The model under review builds one solid part; all positions refer to its coordinate system, in mm. Give positions to 0.01 mm unless a question says otherwise; leave off trailing zeros. Loops run counter-clockwise (first coordinate to the right, second up) from the corner with the lowest first, then second, coordinate; pieces in that order, holes last. Notation, with made-up numbers: M 8.25,-10.5 L 30.25,-10.5 A23 cw 30.25,27.5 Z; hole C 70,-39.5 d9. An arc over 180 degrees is marked long. Return JSON: item names as keys, results as strings.
```python
from build123d import *

# Parameters (mm, degrees)
BOSS_EXTRUDE1_DEPTH = 3.5
SKETCH2_R           = 3.5
SKETCH2_W           = 100
SKETCH2_H           = 40
CUT_EXTRUDE1_DEPTH  = 3.5


with BuildPart() as part:
    # Sketch1 → Boss-Extrude1 (new body)
    with BuildSketch(Plane(origin=(0, 0, 0), x_dir=(1, 0, 0), z_dir=(0, 1, 0))):
        with BuildLine():
            Line((-91.7, 73.2), (91.7, 73.2))
            ThreePointArc((91.7, 73.2), (101.953048327, 68.953048327), (106.2, 58.7))
            Line((106.2, 58.7), (106.2, -58.7))
            ThreePointArc((106.2, -58.7), (101.953048327, -68.953048327), (91.7, -73.2))
            Line((91.7, -73.2), (-91.7, -73.2))
            ThreePointArc((-91.7, -73.2), (-101.953048327, -68.953048327), (-106.2, -58.7))
            Line((-106.2, -58.7), (-106.2, 58.7))
            ThreePointArc((-106.2, 58.7), (-101.953048327, 68.953048327), (-91.7, 73.2))
        make_face()
    extrude(amount=BOSS_EXTRUDE1_DEPTH)

    # Sketch2 → Cut-Extrude1 (cut)
    with BuildSketch(Plane(origin=(0, 3.5, 0), x_dir=(1, 0, 0), z_dir=(0, 1, 0))):
        with Locations(Location((66.2, -26.8, 0), (0, 0, 270))):
            Circle(SKETCH2_R)
        with Locations((36.2, 33.2)):
            Rectangle(SKETCH2_W, SKETCH2_H)
    extrude(amount=-CUT_EXTRUDE1_DEPTH, mode=Mode.SUBTRACT)


solid = part.part
```
1) Wall thickness on L1, parallel to Z at x = -11, y = 3.15; L2, parallel to X at y = 1.35, z = 26.8; L3, parallel to X at y = 3.3, z = -14: over which ranges is each line inside the solid? List them lowest first. Write a range as from..to.
From the geometry:
{"L1": "-73.2..-53.2, -13.2..73.2", "L2": "-106.2..62.7, 69.7..106.2", "L3": "-106.2..-13.8, 86.2..106.2"}
2) The part is to be moulded in two halves that separate along X. For faces 1 (the face through (62.783, 1.774, 26.041)), 2 (the face through (-101.84, 1.726, 69.065)), 3 (the face through (101.84, 1.726, -69.065)), 4 (the face through (1, 0, -1)), say which applies: released by +X, released by -X, zero draft, split by the parting line, or undercut.
From the geometry:
{"face 1": "undercut", "face 2": "released by -X", "face 3": "released by +X", "face 4": "zero draft"}
3) Consider section C-C on x = 66.2. Write out the cut boundary in (y, z), then the cut area to 3 significant figures.
From the geometry:
{"outline": "M 0,-73.2 L 3.5,-73.2 L 3.5,-53.2 L 0,-53.2 Z; M 0,-13.2 L 3.5,-13.2 L 3.5,23.3 L 0,23.3 Z; M 0,30.3 L 3.5,30.3 L 3.5,73.2 L 0,73.2 Z", "area": "348 mm²"}
4) Consider section B-B on z = -22.5. Write out the cut boundary in (x, y), then the cut area to 3 significant figures.
From the geometry:
{"outline": "M -106.2,0 L -13.8,0 L -13.8,3.5 L -106.2,3.5 Z; M 86.2,0 L 106.2,0 L 106.2,3.5 L 86.2,3.5 Z", "area": "393 mm²"}
5) Insertion check: pin 1 (3 mm diameter, centred on x = 15.5, z = -8, fed in from -Y). The pin has a flat end and moves straight along its axis. Give the tip position at first contact, or say it passes through.
From the geometry:
{"pin 1": "y = 0"}
6) Consider section D-D on y = 1.8. Write out the cut boundary in (x, z), then the cut area to 3 significant figures.
From the geometry:
{"outline": "M -106.2,-58.7 A14.5 ccw -91.7,-73.2 L 91.7,-73.2 A14.5 ccw 106.2,-58.7 L 106.2,58.7 A14.5 ccw 91.7,73.2 L -91.7,73.2 A14.5 ccw -106.2,58.7 Z; hole M -13.8,-53.2 L 86.2,-53.2 L 86.2,-13.2 L -13.8,-13.2 Z; hole C 66.2,26.8 d7", "area": "26,900 mm²"}
7) Consider section A-A on x = 4.5. Write out the cut boundary in (y, z), then the cut area to 3 significant figures.
From the geometry:
{"outline": "M 0,-73.2 L 3.5,-73.2 L 3.5,-53.2 L 0,-53.2 Z; M 0,-13.2 L 3.5,-13.2 L 3.5,73.2 L 0,73.2 Z", "area": "372 mm²"}
